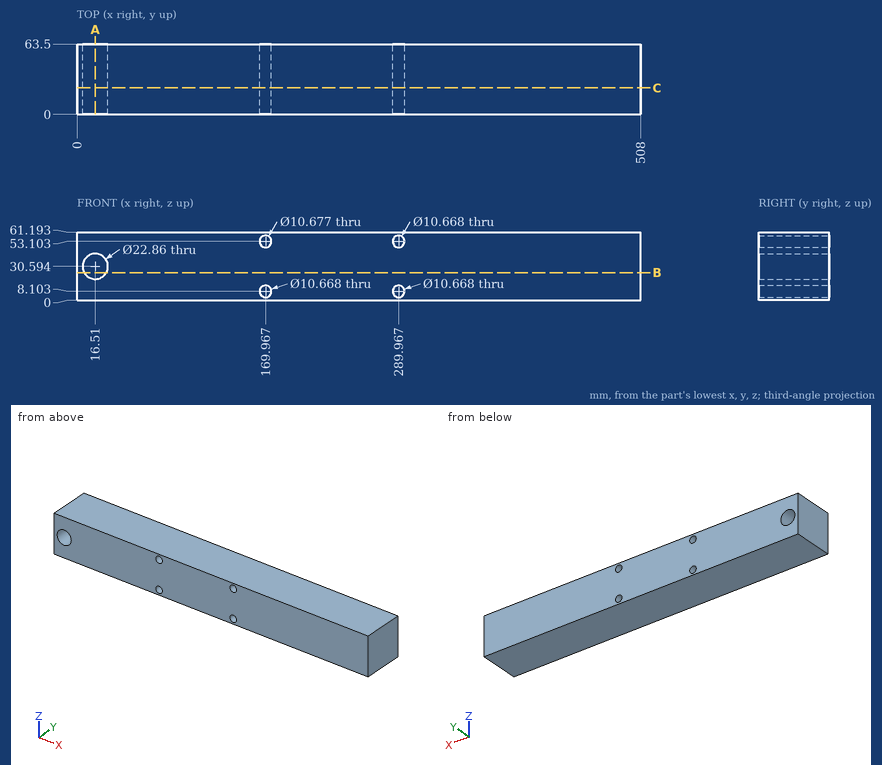
Design review of the part shown in the three views and the two pictorial views. Dimensions are in mm from the part's minimum x, y and z. Round coordinates to 2 decimals unless told otherwise and drop trailing zeros. Order: outer loops, then holes, each group sorted by start corner. A loop starts at its lowest first (then second) coordinate and runs counter-clockwise, first axis right, second up. Notation, with made-up numbers: (49.25, 67) -> (91.25, 67) arc R21 cw to (91.25, 84) -> close; hole circle Ø1 at (1, 6). An arc over 180 degrees is marked (long way). Write item = value, one per line. Start each with the question number.
1) Take a section at B-B on z = 25. State the section outline as (x, y) points.
2) To check wall thickness, follow line 1 (Z direction, x = 290, y = 30); line 2 (X direction, y = 28, z = 54) (1 decimal); line 3 (X direction, y = 49.5, z = 53) (1 decimal). State the ranges of each line that lie inside material, in increasing order. Write a range as from..to.
3) Take a section at C-C on y = 24. State the section outline as (x, z) points (1 decimal), plus the area to 3 significant figures.
4) Take a section at A-A on x = 16.51. State the section outline as (y, z) points (1 decimal).
Verdict:
q1.outline = (0, 0) -> (6.54, 0) -> (6.54, 63.5) -> (0, 63.5) -> close; (26.48, 0) -> (508, 0) -> (508, 63.5) -> (26.48, 63.5) -> close
q2.line_1 = 0..2.77, 13.44..47.77, 58.44..61.19
q2.line_2 = 0..164.7, 175.2..284.7, 295.2..508
q2.line_3 = 0..164.6, 175.3..284.6, 295.3..508
q3.outline = (0, 0) -> (508, 0) -> (508, 61.2) -> (0, 61.2) -> close; hole circle Ø22.9 at (16.5, 30.6); hole circle Ø10.7 at (170, 8.1); hole circle Ø10.7 at (170, 53.1); hole circle Ø10.7 at (290, 8.1); hole circle Ø10.7 at (290, 53.1)
q3.area = 30,300 mm2
q4.outline = (0, 0) -> (63.5, 0) -> (63.5, 19.2) -> (0, 19.2) -> close; (0, 42) -> (63.5, 42) -> (63.5, 61.2) -> (0, 61.2) -> close
